```python
from build123d import *

# Parameters (mm, degrees)
SKETCH1_W                      = 72
SKETCH1_H                      = 67
BASE_FLANGE1_DEPTH             = 0.81
EDGE_FLANGE1_STRIP_W           = 4.7132
EDGE_FLANGE1_STRIP_H           = 0.81
EDGE_FLANGE1_STRIP_CUT_DEPTH   = 72
EDGE_FLANGE1_STRIP_2_W         = 4.7132
EDGE_FLANGE1_STRIP_2_H         = 0.81
EDGE_FLANGE1_STRIP_CUT_2_DEPTH = 72
EDGE_FLANGE1_DEPTH             = 72
EDGE_FLANGE1_BEND_DEPTH        = 72
CUT_EXTRUDE1_REACH             = 148.585
SKETCH12_W                     = 42
SKETCH12_H                     = 30
CUT_EXTRUDE2_REACH             = 148.962
SKETCH13_R                     = 2


# Sheet-metal steps are written as plain solids
with BuildPart() as part:
    # Sketch1 → Base-Flange1 (new body)
    with BuildSketch(Plane(origin=(0, 0, 0), x_dir=(1, 0, 0), z_dir=(0, 1, 0))):
        with Locations((36, 33.5)):
            Rectangle(SKETCH1_W, SKETCH1_H)
    extrude(amount=-BASE_FLANGE1_DEPTH)

    # Edge-Flange1 strip (across the edge) → Edge-Flange1 strip cut (cut)
    with BuildSketch(Plane(origin=(0, 0, 0), x_dir=(0, 0, -1), z_dir=(1, 0, 0))):
        with Locations((-1.62, -0.405)):
            Rectangle(EDGE_FLANGE1_STRIP_W, EDGE_FLANGE1_STRIP_H)
    extrude(amount=EDGE_FLANGE1_STRIP_CUT_DEPTH, mode=Mode.SUBTRACT)

    # Edge-Flange1 strip 2 (across the edge) → Edge-Flange1 strip cut 2 (cut)
    with BuildSketch(Plane(origin=(72, 0, -67), x_dir=(0, 0, 1), z_dir=(-1, 0, 0))):
        with Locations((-1.62, -0.405)):
            Rectangle(EDGE_FLANGE1_STRIP_2_W, EDGE_FLANGE1_STRIP_2_H)
    extrude(amount=EDGE_FLANGE1_STRIP_CUT_2_DEPTH, mode=Mode.SUBTRACT)

    # Edge-Flange1 section (across the edge) → Edge-Flange1 (add)
    with BuildSketch(Plane(origin=(0, 0, 0), x_dir=(0, 0, -1), z_dir=(1, 0, 0))):
        with BuildLine():
            Line((-0.81, 0.7366), (-0.81, 108.19))
            Line((-0.81, 108.19), (0, 108.19))
            Line((0, 108.19), (0, 0.7366))
            ThreePointArc((0, 0.7366), (0.215745145, 0.215745145), (0.7366, 0))
            Line((0.7366, 0), (0.7366, -0.81))
            ThreePointArc((0.7366, -0.81), (-0.357011348, -0.357011348), (-0.81, 0.7366))
        make_face()
    extrude(amount=EDGE_FLANGE1_DEPTH)

    # Edge-Flange1 section 2 (across the edge) → Edge-Flange1 bend (add)
    with BuildSketch(Plane(origin=(72, 0, -67), x_dir=(0, 0, 1), z_dir=(-1, 0, 0))):
        with BuildLine():
            Line((-0.81, 0.7366), (-0.81, 108.19))
            Line((-0.81, 108.19), (0, 108.19))
            Line((0, 108.19), (0, 0.7366))
            ThreePointArc((0, 0.7366), (0.215745145, 0.215745145), (0.7366, 0))
            Line((0.7366, 0), (0.7366, -0.81))
            ThreePointArc((0.7366, -0.81), (-0.357011348, -0.357011348), (-0.81, 0.7366))
        make_face()
    extrude(amount=EDGE_FLANGE1_BEND_DEPTH)

    # Sketch12 → Cut-Extrude1 (cut, up to next)
    with BuildSketch(Plane(origin=(0, 0, 0), x_dir=(1, 0, 0), z_dir=(0, 1, 0)), mode=Mode.PRIVATE) as cut_extrude1_sk1:
        with Locations((36, 33.5)):
            Rectangle(SKETCH12_W, SKETCH12_H)
    cut_extrude1_tool1 = extrude(cut_extrude1_sk1.sketch, amount=-CUT_EXTRUDE1_REACH, mode=Mode.PRIVATE) & part.part
    add(cut_extrude1_tool1.solids().sort_by_distance((36, 0, -33.5))[0], mode=Mode.SUBTRACT)

    # Cut-Extrude2: up to this face of the body (flat: up to its plane)
    cut_extrude2_end = Plane(part.part.faces().sort_by_distance((36, 54.4633, 0.81))[0])
    # Sketch13 → Cut-Extrude2 (cut, up to the picked face)
    with BuildSketch(Plane(origin=(0, 0, -67.81), x_dir=(-1, 0, 0), z_dir=(0, 0, -1)), mode=Mode.PRIVATE) as cut_extrude2_sk1:
        with Locations(Location((-9, 52.1466, 0), (0, 0, 90))):
            Circle(SKETCH13_R)
    cut_extrude2_tool1 = split(extrude(cut_extrude2_sk1.sketch, amount=-CUT_EXTRUDE2_REACH, mode=Mode.PRIVATE), bisect_by=cut_extrude2_end, keep=Keep.BOTH, mode=Mode.PRIVATE)
    # Sketch13 → Cut-Extrude2 (cut, up to the picked face)
    with BuildSketch(Plane(origin=(0, 0, -67.81), x_dir=(-1, 0, 0), z_dir=(0, 0, -1)), mode=Mode.PRIVATE) as cut_extrude2_sk2:
        with Locations(Location((-60, 52.1466, 0), (0, 0, 90))):
            Circle(SKETCH13_R)
    cut_extrude2_tool2 = split(extrude(cut_extrude2_sk2.sketch, amount=-CUT_EXTRUDE2_REACH, mode=Mode.PRIVATE), bisect_by=cut_extrude2_end, keep=Keep.BOTH, mode=Mode.PRIVATE)
    add(cut_extrude2_tool1.solids().sort_by(Axis((9, 52.1466, -67.81), (0, 0, 1)))[0], mode=Mode.SUBTRACT)
    add(cut_extrude2_tool2.solids().sort_by(Axis((60, 52.1466, -67.81), (0, 0, 1)))[0], mode=Mode.SUBTRACT)


solid = part.part
```
Read the model definition and answer for the solid it produces. Units are mm, in the model's axes. A direction names the side the tool comes from. Give positions to 0.01 mm unless a question says otherwise; leave off trailing zeros. Order: outer loops, then holes, each group sorted by start corner. A loop starts at its lowest first (then second) coordinate and runs counter-clockwise, first axis right, second up.
(1) For a pull along Y with two mould halves and no side action, classify faces 3 (the flat face through (35, -0.81, -49)), 4 (the cylindrical face through (9.601, 54.054, 0.399)), 5 (the flat face through (35, 55, 0)) as released by +Y, released by -Y, zero draft, split by the parting line, or undercut.
(2) Find section D-D (z = -22). Give the vertices of the cut face in (x, y).
(3) Find section A-A (x = 60). Give the vertices of the cut face in (y, z), plus the area to 3 significant figures.
(4) Given pin 1 (19.5 mm diameter, centred on x = 50.5, z = -33.5, fed in from +Y); pin 2 (0.6 mm diameter, centred on x = 37.5, y = -0.5, fed in from -Z); pin 3 (0.9 mm diameter, centred on x = 29.5, y = -0.5, fed in from +Z) (3 decimals), each flat-ended and moving along its own axis, determine where each tip first touches the part or whether it passes through.
(5) For faces 1 (the flat face through (35, 54, 0.81)), 2 (the flat face through (35, 0, -49)), determine the directions among +Z, -Z, +X, -X, +Y, -Y from which every point of the face is accessible in a straight line to the end or side of a thin tool.
(6) Find section C-C (y = 81). Give the vertices of the cut face in (x, z).
(7) Straight lines are drawn through the part: L1, parallel to Z at x = 35, y = 32; L2, parallel to Y at x = 29.5, z = -17. For each, find the intervals that lie inside material, in ascending order.
(8) Find section B-B (x = 52). Give the vertices of the cut face in (y, z), plus the area to 3 significant figures.
Result sheet:
1. face 3: released by -Y
1. face 4: undercut
1. face 5: zero draft
2. outline: (0, -0.81) - (15, -0.81) - (15, 0) - (0, 0) - close; (57, -0.81) - (72, -0.81) - (72, 0) - (57, 0) - close
3. outline: (-0.81, -66.26) arc R1.55 ccw to (0.74, -67.81) - (50.15, -67.81) - (50.15, -67) - (0.74, -67) arc R0.74 cw to (0, -66.26) - (0, -0.74) arc R0.74 cw to (0.74, 0) - (50.15, 0) - (50.15, 0.81) - (0.74, 0.81) arc R1.55 ccw to (-0.81, -0.74) - close; (54.15, -67.81) - (108.19, -67.81) - (108.19, -67) - (54.15, -67) - close; (54.15, 0) - (108.19, 0) - (108.19, 0.81) - (54.15, 0.81) - close
3. area: 224 mm2
4. pin 1: stops at y = 0
4. pin 2: stops at z = -67.49
4. pin 3: stops at z = 0.595
5. face 1: +Z, +X, -X, +Y, -Y
5. face 2: +X, -X, +Y
6. outline: (0, -67.81) - (72, -67.81) - (72, -67) - (0, -67) - close; (0, 0) - (72, 0) - (72, 0.81) - (0, 0.81) - close
7. L1: z = -67.81 to -67, 0 to 0.81
7. L2: y = -0.81 to 0
8. outline: (-0.81, -66.26) arc R1.55 ccw to (0.74, -67.81) - (108.19, -67.81) - (108.19, -67) - (0.74, -67) arc R0.74 cw to (0, -66.26) - (0, -48.5) - (-0.81, -48.5) - close; (-0.81, -18.5) - (0, -18.5) - (0, -0.74) arc R0.74 cw to (0.74, 0) - (108.19, 0) - (108.19, 0.81) - (0.74, 0.81) arc R1.55 ccw to (-0.81, -0.74) - close
8. area: 206 mm2
